from build123d import *

# Parameters (mm, degrees)
F2_SIZE  = 0.5
F3_R     = 5
F3_R_2   = 3.9
F4_DEPTH = 0.4
F5_R     = 2
F6_R     = 1.6
F7_DEPTH = 25
F8_R     = 1.6
F9_DEPTH = 2.5


with BuildPart() as f1:
    # F0 (on Front) → F1 (revolve)
    with BuildSketch(Plane.XZ):
        Polygon((3.9, 6), (0, 6), (0, 0), (10, 0), (10, 3), (3.9, 3), align=None)
    revolve(axis=Axis((0, 0, 3), (0, 0, -1)))

    # F2
    f2_edges = [f1.edges().sort_by_distance(p)[0] for p in [
        (-3.9, 0, 6),
    ]]
    chamfer(f2_edges, length=F2_SIZE)

    # F3 (on face) → F4 (join)
    with BuildSketch(Plane.XY.offset(3)):
        Circle(F3_R)
        Circle(F3_R_2, mode=Mode.SUBTRACT)
    extrude(amount=F4_DEPTH)

    # F5
    f5_edges = [f1.edges().sort_by_distance(p)[0] for p in [
        (-10, 0, 0),
    ]]
    fillet(f5_edges, radius=F5_R)

    # F6 (on face) → F7 (cut)
    with BuildSketch(Plane.XY.offset(6)):
        Circle(F6_R)
    extrude(amount=-F7_DEPTH, mode=Mode.SUBTRACT)

    # F8 (on face) → F9 (cut)
    with BuildSketch(Plane(origin=(0, 0, 0), x_dir=(1, 0, 0), z_dir=(0, 0, -1))):
        Polygon((3, -1.732051), (3, 1.732051), (0, 3.464102), (-3, 1.732051), (-3, -1.732051), (0, -3.464102), align=None)
        Circle(F8_R, mode=Mode.SUBTRACT)
    extrude(amount=-F9_DEPTH, mode=Mode.SUBTRACT)


solid = f1.part
Read the model definition and answer for the solid it produces. Units are mm, in the model's axes. A direction names the side the tool comes from. Coordinates: 2 decimals unless noted, no trailing zeros. Order: outer loops, then holes, each group sorted by start corner. A loop starts at its lowest first (then second) coordinate and runs counter-clockwise, first axis right, second up. Notation, with made-up numbers: M 66.25,-32.5 L 96.25,-32.5 A21 ccw 96.25,-23.5 Z; hole C -1.75,2 d6. An arc over 180 degrees is marked long. Put each result on its own line as item: value. Start each with the question number.
Item 1: For faces 4 (the face through (-2, 1, 6)), 5 (the face through (-1.5, -2.6, 1.2)), 6 (the face through (-2.87, -2.64, 4.46)), determine the directions among +Z, -Z, +X, -X, +Y, -Y from which every point of the face is accessible in a straight line to the end or side of a thin tool.
Item 2: Section B-B, the plane z = 0.85 is taken. Determine the outline of the cut face in (x, y), plus the area to 3 significant figures.
Item 3: Given pin 1 Ø0.8 at (y, z) = (1, 1) entering from +X; pin 2 Ø1.5 at (y, z) = (-5, 3.5) entering from -X; pin 3 Ø3 at (x, y) = (0, 0) entering from +Z; pin 4 Ø1 at (y, z) = (0, 4) entering from +X, each flat-ended and moving along its own axis, determine where each tip first touches the part or whether it passes through.
Item 4: The mould has two halves that part along Y. Classify faces 1 (the face through (-2.17, 9.76, 2.51)), 2 (the face through (-3, 0, 1)), 3 (the face through (2, -5, 3)): +Y half, -Y half, draft (parallel to the pull), parting line (faces both ways), or undercut.
Item 5: Consider probe 1 along Y at (x, z) = (0, 5); probe 2 along Z at (x, y) = (-7.75, 0). Determine where each line is inside the solid, lowest interval first. Write a range as [from, to].
Item 6: Section A-A, the plane y = 0 is taken. Determine the outline of the cut face in (x, z), plus the area to 3 significant figures.
Computed:
1. face 4: +Z, +X, -X, +Y, -Y
1. face 5: -Z
1. face 6: +Z
2. outline: C 0,0 d19.27; hole M -3,-1.73 L 0,-3.46 L 3,-1.73 L 3,1.73 L 0,3.46 L -3,1.73 Z
2. area: 261 mm2
3. pin 1: stops at x = 9.86
3. pin 2: stops at x = -8.96
3. pin 3: passes through
3. pin 4: stops at x = 3.9
4. face 1: parting line
4. face 2: undercut
4. face 3: draft
5. probe 1: y = [-3.9, -1.6], [1.6, 3.9]
5. probe 2: z = [0, 3]
6. outline: M -10,2 A2 ccw -8,0 L -3,0 L -3,2.5 L -1.6,2.5 L -1.6,6 L -3.4,6 L -3.9,5.5 L -3.9,3.4 L -5,3.4 L -5,3 L -10,3 Z; M 1.6,2.5 L 3,2.5 L 3,0 L 8,0 A2 ccw 10,2 L 10,3 L 5,3 L 5,3.4 L 3.9,3.4 L 3.9,5.5 L 3.4,6 L 1.6,6 Z
6. area: 56.1 mm2
